The listing builds one solid part. Answer for the finished solid, in the listing's coordinates (mm). A direction names the side the tool comes from. Round coordinates to 2 decimals unless told otherwise and drop trailing zeros. Write each loop counter-clockwise with the first axis right and the second up, starting at its lowest first coordinate (ties: lowest second). Pieces come first, ordered by that corner, then holes. Notation, with made-up numbers: (28, 1) - (65, 1) arc R30 cw to (65, 23) - close; hole circle Ø5 at (32, 61). An arc over 180 degrees is marked (long way). Answer in a Markdown table with one row per item.
from build123d import *

# Parameters (mm, degrees)
SKETCH_1_W                  = 82
SKETCH_1_H                  = 63.5
EXTRUDE_1_DEPTH             = 16
CUT_EXTRUDE_1_DEPTH         = 83
SKETCH_15_W                 = 23.6
SKETCH_15_H                 = 14.711451884
CUT_EXTRUDE_4_DEPTH         = 7
SKETCH_16_W                 = 23.6
SKETCH_16_H                 = 10.67
CUT_EXTRUDE_5_DEPTH         = 9
SKETCH_17_R                 = 2.5
CUT_EXTRUDE_6_DEPTH         = 8
M4X0_72_D                   = 3.3
M4X0_72_DEPTH               = 10
M4X0_72_TIP                 = 0.991420021
CUT_EXTRUDE_7_DEPTH         = 4
SKETCH_26_R                 = 3.25
CUT_EXTRUDE_8_DEPTH         = 38
HOLE_WIZARD_M41_D           = 4.5
HOLE_WIZARD_M41_CBORE_D     = 8
HOLE_WIZARD_M41_CBORE_DEPTH = 4
CHAMFER_2_SIZE              = 1
CHAMFER_2_SIZE2             = 2
CHAMFER_2_PART_2_SIZE       = 1
CHAMFER_2_PART_2_SIZE2      = 2
CHAMFER_2_PART_3_SIZE       = 1
CHAMFER_2_PART_3_SIZE2      = 2
CUT_EXTRUDE_12_DEPTH        = 10.6
FILLET_1_R                  = 3
M4X0_73_D                   = 3.3


with BuildPart() as part:
    # Эскиз1 → Бобышка-Вытянуть1 (new body)
    with BuildSketch(Plane.XY):
        with Locations((41, -31.75)):
            Rectangle(SKETCH_1_W, SKETCH_1_H)
    extrude(amount=EXTRUDE_1_DEPTH)

    # Эскиз2 → Вырез-Вытянуть1 (cut, through all)
    with BuildSketch(Plane.ZY):
        Polygon((9, -10.67), (16, -14.711451884), (16, -48.788548116), (9, -52.83), align=None)
    extrude(amount=-CUT_EXTRUDE_1_DEPTH, mode=Mode.SUBTRACT)

    # Эскиз15 → Вырез-Вытянуть4 (cut)
    with BuildSketch(Plane.XY.offset(16)):
        with Locations((41, -56.144274058)):
            Rectangle(SKETCH_15_W, SKETCH_15_H)
    extrude(amount=-CUT_EXTRUDE_4_DEPTH, mode=Mode.SUBTRACT)

    # Эскиз16 → Вырез-Вытянуть5 (cut)
    with BuildSketch(Plane.XY.offset(9)):
        with Locations((41, -58.165)):
            Rectangle(SKETCH_16_W, SKETCH_16_H)
    extrude(amount=-CUT_EXTRUDE_5_DEPTH, mode=Mode.SUBTRACT)

    # Эскиз17 → Вырез-Вытянуть6 (cut)
    with BuildSketch(Plane.XZ.offset(52.83)):
        with Locations((33.5, 5)):
            Circle(SKETCH_17_R)
        with Locations((48.5, 5)):
            Circle(SKETCH_17_R)
    extrude(amount=-CUT_EXTRUDE_6_DEPTH, mode=Mode.SUBTRACT)

    # Отверстие обработанное метчиком M4x0.72
    with Locations(Plane(origin=(0, -52.83, 0), x_dir=(-1, 0, 0), z_dir=(0, -1, 0))):
        with Locations((-41, -5)):
            Hole(M4X0_72_D / 2, depth=M4X0_72_DEPTH)
            with Locations((0, 0, -(M4X0_72_DEPTH + M4X0_72_TIP / 2))):  # 118° drill point
                Cone(0, M4X0_72_D / 2, M4X0_72_TIP, mode=Mode.SUBTRACT)

    # Эскиз25 → Вырез-Вытянуть7 (cut)
    with BuildSketch(Plane.XY.offset(9)):
        with BuildLine():
            Line((44.1, -18.711451884), (44.1, -25.711451884))
            ThreePointArc((44.1, -25.711451884), (41, -28.811451884), (37.9, -25.711451884))
            Line((37.9, -25.711451884), (37.9, -18.711451884))
            ThreePointArc((37.9, -18.711451884), (41, -15.611451884), (44.1, -18.711451884))
        make_face()
    extrude(amount=-CUT_EXTRUDE_7_DEPTH, mode=Mode.SUBTRACT)

    # Эскиз26 → Вырез-Вытянуть8 (cut)
    with BuildSketch(Plane(origin=(0, 0, 0), x_dir=(1, 0, 0), z_dir=(0, 1, 0))):
        with Locations((41, -4.5)):
            Circle(SKETCH_26_R)
    extrude(amount=-CUT_EXTRUDE_8_DEPTH, mode=Mode.SUBTRACT)

    # Цековка для винта с внутренним шестигранником M41 (through all)
    with Locations(Plane(origin=(30.759227947, 26.793365177, 16), x_dir=(-1, 0, 0), z_dir=(0, 0, 1))):
        with Locations((-46.240772053, 31.793365177), (-46.240772053, 85.293365177), (25.759227947, 85.293365177), (25.759227947, 31.793365177)):
            CounterBoreHole(HOLE_WIZARD_M41_D / 2, HOLE_WIZARD_M41_CBORE_D / 2, HOLE_WIZARD_M41_CBORE_DEPTH)

    # Фаска2
    chamfer_2_edges = [part.edges().sort_by_distance(p)[0] for p in [
        (41, -14.711451884, 16),
    ]]
    chamfer_2_side = [part.faces().sort_by_distance(p)[0] for p in [
        (41, -7.569889145, 16),
    ]]
    chamfer(chamfer_2_edges, length=CHAMFER_2_SIZE, length2=CHAMFER_2_SIZE2, reference=chamfer_2_side[0])

    # Фаска2 part 2
    chamfer_2_part_2_edges = [part.edges().sort_by_distance(p)[0] for p in [
        (67.4, -48.788548116, 16),
    ]]
    chamfer_2_part_2_side = [part.faces().sort_by_distance(p)[0] for p in [
        (66.127821531, -55.832096576, 16),
    ]]
    chamfer(chamfer_2_part_2_edges, length=CHAMFER_2_PART_2_SIZE, length2=CHAMFER_2_PART_2_SIZE2, reference=chamfer_2_part_2_side[0])

    # Фаска2 part 3
    chamfer_2_part_3_edges = [part.edges().sort_by_distance(p)[0] for p in [
        (14.6, -48.788548116, 16),
    ]]
    chamfer_2_part_3_side = [part.faces().sort_by_distance(p)[0] for p in [
        (15.872178469, -55.832096576, 16),
    ]]
    chamfer(chamfer_2_part_3_edges, length=CHAMFER_2_PART_3_SIZE, length2=CHAMFER_2_PART_3_SIZE2, reference=chamfer_2_part_3_side[0])

    # Эскиз32 → Вырез-Вытянуть12 (cut)
    with BuildSketch(Plane.XZ.offset(63.5)):
        with BuildLine():
            Line((52.7, -0.2), (52.7, 3.7))
            Line((52.7, 3.7), (58.5, 3.7))
            ThreePointArc((58.5, 3.7), (62.8, 8), (58.5, 12.3))
            Line((58.5, 12.3), (52.7, 12.3))
            Line((52.7, 12.3), (52.7, 16.2))
            Line((52.7, 16.2), (29.3, 16.2))
            Line((29.3, 16.2), (29.3, 12.3))
            Line((29.3, 12.3), (23.5, 12.3))
            ThreePointArc((23.5, 12.3), (19.2, 8), (23.5, 3.7))
            Line((23.5, 3.7), (29.3, 3.7))
            Line((29.3, 3.7), (29.3, -0.2))
            Line((29.3, -0.2), (52.7, -0.2))
        make_face()
    extrude(amount=-CUT_EXTRUDE_12_DEPTH, mode=Mode.SUBTRACT)

    # Скругление1
    fillet_1_edges = [part.edges().sort_by_distance(p)[0] for p in [
        (52.8, -58.2, 3.7),
        (52.8, -58.2, 12.3),
        (29.2, -58.2, 12.3),
        (29.2, -58.2, 3.7),
    ]]
    fillet(fillet_1_edges, radius=FILLET_1_R)

    # Отверстие обработанное метчиком M4x0.73 (through all)
    with Locations(Plane(origin=(0, 0, 0), x_dir=(-1, 0, 0), z_dir=(0, 0, -1))):
        with Locations((-26, -44.75), (-26, -18.75), (-56, -18.75), (-56, -44.75)):
            Hole(M4X0_73_D / 2)


solid = part.part
(1) Section C-C (x = 64) is taken. Give the vertices of the cut face in (y, z).
Checked values:
| item | result |
|---|---|
| outline | (-63.5, 0) - (0, 0) - (0, 16) - (-13.71, 16) - (-13.71, 14.27) - (-10.67, 9) - (-52.83, 9) - (-49.79, 14.27) - (-49.79, 16) - (-63.5, 16) - close |
(2) Section D-D (x = 48.5) is taken. Give the vertices of the cut face in (y, z).
Checked values:
| item | result |
|---|---|
| outline | (-52.83, 0) - (0, 0) - (0, 16) - (-13.71, 16) - (-13.71, 14.27) - (-10.67, 9) - (-52.83, 9) - (-52.83, 7.5) - (-44.83, 7.5) - (-44.83, 2.5) - (-52.83, 2.5) - close |
(3) Section A-A (y = -5) is taken. Give the vertices of the cut face in (x, z), and give its area (3 significant figures).
Checked values:
| item | result |
|---|---|
| outline | (0, 0) - (2.75, 0) - (2.75, 12) - (1, 12) - (1, 16) - (0, 16) - close; (7.25, 0) - (74.75, 0) - (74.75, 12) - (73, 12) - (73, 16) - (9, 16) - (9, 12) - (7.25, 12) - close; (79.25, 0) - (82, 0) - (82, 16) - (81, 16) - (81, 12) - (79.25, 12) - close; hole circle Ø6.5 at (41, 4.5) |
| area | 1,110 mm2 |
(4) Find the intervals of material crossed by line 1 (Y direction, x = 5, z = 2.75); line 2 (X direction, y = -58.5, z = 9.25); line 3 (Y direction, x = 56, z = 6.75), in increasing order.
Checked values:
| item | result |
|---|---|
| line 1 | y = -63.5 to -60.75, -56.25 to -7.25, -2.75 to 0 |
| line 2 | x = 0 to 2.75, 7.25 to 19.39, 62.61 to 74.75, 79.25 to 82 |
| line 3 | y = -52.9 to -46.4, -43.1 to -20.4, -17.1 to 0 |
(5) Flat-ended cylindrical pins translate along their axes: pin 1 (5.5 mm diameter, centred on x = 56, y = -18.75, fed in from +Z); pin 2 (4.5 mm diameter, centred on x = 33.5, z = 5, fed in from -Y); pin 3 (6.5 mm diameter, centred on x = 48.5, z = 5, fed in from -Y); pin 4 (2.5 mm diameter, centred on x = 77, y = -58.5, fed in from +Z). Find the tip coordinate at first contact, or state that the pin passes through.
Checked values:
| item | result |
|---|---|
| pin 1 | stops at z = 9 |
| pin 2 | stops at y = -44.83 |
| pin 3 | stops at y = -52.83 |
| pin 4 | passes through |
(6) For a pull along Y with two mould halves and no side action, classify faces 1 (the flat face through (40, -32, 9)), 2 (the cylindrical face through (53.66, -58.13, 2.8)), 3 (the flat face through (33, -44.83, 5)), 4 (the flat face through (44.1, -22, 7)) as pulls with the +Y half, pulls with the -Y half, needs draft (parallel to the pull), parting line crosses it, or undercut.
Checked values:
| item | result |
|---|---|
| face 1 | undercut |
| face 2 | needs draft |
| face 3 | pulls with the -Y half |
| face 4 | undercut |
(7) Section B-B (x = 77) is taken. Give the vertices of the cut face in (y, z), and give its area (3 significant figures).
Checked values:
| item | result |
|---|---|
| outline | (-63.5, 0) - (-60.75, 0) - (-60.75, 12) - (-62.5, 12) - (-62.5, 16) - (-63.5, 16) - close; (-56.25, 0) - (-7.25, 0) - (-7.25, 12) - (-9, 12) - (-9, 16) - (-13.71, 16) - (-13.71, 14.27) - (-10.67, 9) - (-52.83, 9) - (-49.79, 14.27) - (-49.79, 16) - (-54.5, 16) - (-54.5, 12) - (-56.25, 12) - close; (-2.75, 0) - (0, 0) - (0, 16) - (-1, 16) - (-1, 12) - (-2.75, 12) - close |
| area | 575 mm2 |
(8) For faces 5 (the cylindrical face through (41.07, -28.81, 8.05)), 6 (the flat face through (48, -44.83, 5)), 7 (the flat face through (67, -49.789, 15)), 8 (the flat face through (41, -52.83, 3)), determine the directions among +Z, -Z, +X, -X, +Y, -Y from which every point of the face is accessible in a straight line to the end or side of a thin tool.
Checked values:
| item | result |
|---|---|
| face 5 | +Z |
| face 6 | -Y |
| face 7 | +Z, +X, -X |
| face 8 | +Z, -Z, -Y |
